Source: CAD feature listing. Evaluate the final solid. Frame: model axes, mm. A direction names the side the tool comes from. Coordinates: 2 decimals unless noted, no trailing zeros. Write each loop counter-clockwise with the first axis right and the second up, starting at its lowest first coordinate (ties: lowest second). Pieces come first, ordered by that corner, then holes. Notation, with made-up numbers: (13.5, 38.25) -> (64.5, 38.25) arc R23 cw to (64.5, 70.25) -> close; hole circle Ø9 at (40, -17.5). An arc over 180 degrees is marked (long way). One line per item, written item: value. Start each with the question number.
1. First-contact query: P1, Ø2.5, axis at y = -9, z = 2, coming from the +X side; P2, Ø20, axis at x = -35.5, y = -6.5, coming from the +Z side; P3, Ø6, axis at x = -46.5, y = -8.5, coming from the +Z side. Flat tips, straight axial feed; report the tip coordinate or a pass-through.
2. Access query for faces 4 (the flat face through (-52.64, -8.28, 27.6)), 5 (the flat face through (-39, -1, 10)), 6 (the flat face through (-39, -1, 5)). Directions: +Z, -Z, +X, -X, +Y, -Y. A direction counts if a zero-diameter tool reaches every point of the face in a straight line with its end or side. Return the directions, or none.
3. Section query B-B, the plane x = -4. Output: boundary loops of the cut face in (y, z).
4. Mould query, pull axis X, two halves, no side actions, for faces 1 (the flat face through (-53, 4, 35)), 2 (the flat face through (-47.57, -3, 20)), 3 (the cylindrical face through (-8.65, 11.51, 10.12)). Classes: released by +X, released by -X, zero draft, split by the parting line, or undercut.
5. Section query A-A, the plane z = 15. Output: boundary loops of the cut face in (x, y).
6. Line query: line 1 (Y direction, x = -29.5, z = 28); line 2 (Z direction, x = -32, y = 6); line 3 (X direction, y = -12.5, z = 24). Output: solid intervals per line, ascending.
7. Section query C-C, the plane y = 5.5. Output: boundary loops of the cut face in (x, z).
8. Section query D-D, the plane x = -11. Output: boundary loops of the cut face in (y, z).
from build123d import *

# Parameters (mm, degrees)
F0_W      = 65
F0_H      = 35
F1_DEPTH  = 40
F2_W      = 10
F2_H      = 5
F3_DEPTH  = 5
F5_DEPTH  = 65
F6_DEPTH  = 65
F7_W      = 25
F7_H      = 5
F8_DEPTH  = 55
F10_DEPTH = 25
F12_DEPTH = 25
F13_R     = 5
F14_DEPTH = 25


with BuildPart() as f1:
    # F0 (on Top) → F1 (new body)
    with BuildSketch(Plane.XY):
        with Locations((-25.0700588524, -0.9162277728)):
            Rectangle(F0_W, F0_H)
    extrude(amount=F1_DEPTH)

    # F2 (on face) → F3 (cut)
    with BuildSketch(Plane.XY.offset(40)):
        with Locations((-52.5700588524, 4.0837722272)):
            Rectangle(F2_W, F2_H)
    extrude(amount=-F3_DEPTH, mode=Mode.SUBTRACT)

    # F4 (on face) → F5 (cut)
    with BuildSketch(Plane(origin=(-57.5700588524, 0, 0), x_dir=(0, -1, 0), z_dir=(-1, 0, 0))):
        Polygon((-1.5837722272, 40), (-1.5837722272, 35), (18.4162277728, 20), (18.4162277728, 40), align=None)
    extrude(amount=-F5_DEPTH, mode=Mode.SUBTRACT)

    # F6 (cut): a face of the model
    f6_faces = [f1.faces().sort_by_distance(p)[0] for p in [
        (-47.5700588524, 4.0837722272, 37.5),
    ]]
    extrude(f6_faces, amount=-F6_DEPTH, mode=Mode.SUBTRACT)

    # F7 (on face) → F8 (cut)
    with BuildSketch(Plane.YZ.offset(7.4299411476)):
        Polygon((6.5837722272, 10), (6.5837722272, 35), (1.5837722272, 35), (-18.4162277728, 20), (-18.4162277728, 10), align=None)
        with Locations((-5.9162277728, 2.5)):
            Rectangle(F7_W, F7_H)
    extrude(amount=-F8_DEPTH, mode=Mode.SUBTRACT)

    # F9 (on face) → F10 (cut)
    with BuildSketch(Plane(origin=(0, 16.5837722272, 0), x_dir=(-1, 0, 0), z_dir=(0, 1, 0))):
        Polygon((-7.4299411476, 20), (32.5700588524, 40), (-7.4299411476, 40), align=None)
    extrude(amount=-F10_DEPTH, mode=Mode.SUBTRACT)

    # F11 (on face) → F12 (cut)
    with BuildSketch(Plane.XY.offset(10)):
        Polygon((-17.5700588524, 6.5837722272), (-47.5700588524, -18.4162277728), (7.4299411476, -18.4162277728), (7.4299411476, 6.5837722272), align=None)
    extrude(amount=-F12_DEPTH, mode=Mode.SUBTRACT)

    # F13 (on face) → F14 (cut)
    with BuildSketch(Plane.XZ.offset(-6.5837722272)):
        with Locations((-7.5700588524, 15)):
            Circle(F13_R)
    extrude(amount=-F14_DEPTH, mode=Mode.SUBTRACT)


solid = f1.part
Computed values:
1. P1: stops at x = -47.57
1. P2: stops at z = 10
1. P3: stops at z = 29.54
2. face 4: +Z, +X, -X, -Y
2. face 5: +Z, +X, -Y
2. face 6: -Z, +X, -Y
3. outline: (6.58, 0) -> (16.58, 0) -> (16.58, 11.5) -> (6.58, 11.5) -> close; (6.58, 18.5) -> (16.58, 18.5) -> (16.58, 25.71) -> (6.58, 25.71) -> close
4. face 1: zero draft
4. face 2: released by +X
4. face 3: undercut
5. outline: (-57.57, -18.42) -> (-47.57, -18.42) -> (-47.57, 6.58) -> (-12.57, 6.58) -> (-12.57, 16.58) -> (-57.57, 16.58) -> close; (-2.57, 6.58) -> (7.43, 6.58) -> (7.43, 16.58) -> (-2.57, 16.58) -> close
6. line 1: y = 6.58 to 16.58
6. line 2: z = 5 to 10
6. line 3: x = -57.57 to -47.57
7. outline: (-57.57, 0) -> (-47.57, 0) -> (-47.57, 5) -> (-18.87, 5) -> (-18.87, 10) -> (-47.57, 10) -> (-47.57, 35) -> (-57.57, 35) -> close
8. outline: (6.58, 0) -> (16.58, 0) -> (16.58, 11.36) -> (6.58, 11.36) -> close; (6.58, 18.64) -> (16.58, 18.64) -> (16.58, 29.21) -> (6.58, 29.21) -> close
